Design review of the part built by this model. Coordinates are the model's own, in mm. A direction names the side the tool comes from. Coordinates: 2 decimals unless noted, no trailing zeros. Write each loop counter-clockwise with the first axis right and the second up, starting at its lowest first coordinate (ties: lowest second). Pieces come first, ordered by that corner, then holes.
Q1. For L1, parallel to Y at x = 37, z = 4.75; L2, parallel to Z at x = 2.5, y = 39; L3, parallel to X at y = 6.5, z = 3.25, list the stretches that pass through material, from the lowest coordinate up.
Q2. For faces 3 (the cylindrical face through (28, 9.1, 14)), 4 (the flat face through (36, 22, 13)), list the 3-axis set-ups (+Z, -Z, +X, -X, +Y, -Y) from which the entire face can be reached by the end or side of a thin tool; tool diameter is ignored.
Q3. The part is to be moulded in two halves that separate along Z. For faces 1 (the flat face through (21, 36, 2)), 2 (the flat face through (43, 22, 14)), say which applies: released by +Z, released by -Z, zero draft, split by the parting line, or undercut.
Q4. Take a section at C-C, the plane x = 37. Write out the cut boundary in (y, z).
Q5. For pin 1 Ø22.5 at (x, y) = (21.5, 21.5) entering from +Z, flat-tipped, find the tip position at first contact; note if it passes through.
Q6. Take a section at B-B, the plane x = 21.5. Write out the cut boundary in (y, z), plus the area to 3 significant figures.
Q7. Take a section at A-A, the plane z = 5.5. Write out the cut boundary in (x, y).
Solid Edge part; units mm, degrees
sketch "Sketch1" plane through (0, 0, 0) normal (0, 0, 1) x (1, 0, 0)
  line L0 (7, 0) -> (36, 0)
  arc A0 (36, 0) -> (43, 7) centre (36, 7) ccw
  line L1 (43, 7) -> (43, 36)
  arc A1 (43, 36) -> (36, 43) centre (36, 36) ccw
  line L2 (36, 43) -> (7, 43)
  arc A2 (7, 43) -> (0, 36) centre (7, 36) ccw
  line L3 (0, 36) -> (0, 7)
  arc A3 (7, 0) -> (0, 7) centre (7, 7) cw
  circle A4 centre (21.5, 21.5) radius 14
  circle A5 centre (6, 37) radius 1.7
  circle A6 centre (37, 37) radius 1.7
  circle A7 centre (6, 6) radius 1.7
  circle A8 centre (37, 6) radius 1.7
extrude "Protrusion1" add sketch "Sketch1" along normal blind 2
sketch "Sketch2" plane through (21.5, 21.5, 2) normal (0, 0, 1) x (1, 0, 0)
  circle A0 centre (-15.5, -15.5) radius 3.5
  circle A1 centre (-15.5, 15.5) radius 3.5
  circle A2 centre (15.5, 15.5) radius 3.5
  circle A3 centre (15.5, -15.5) radius 3.5
  circle A4 centre (-15.5, 15.5) radius 1.7
  circle A5 centre (15.5, 15.5) radius 1.7
  circle A6 centre (-15.5, -15.5) radius 1.7
  circle A7 centre (15.5, -15.5) radius 1.7
extrude "ExtrudedProtrusion_2" add sketch "Sketch2" along normal blind 11
mirror "Mirror1" about plane through (21.5, 21.5, 7.5) normal (0, 0, -1) of "Protrusion1"
Responses:
1. L1: y = 2.5 to 4.3, 7.7 to 9.5, 33.5 to 35.3, 38.7 to 40.5
1. L2: z = 0 to 2, 13 to 15
1. L3: x = 2.54 to 4.38, 7.62 to 9.46, 33.54 to 35.38, 38.62 to 40.46
2. face 3: +Z, -Z
2. face 4: none
3. face 1: undercut
3. face 2: zero draft
4. outline: (0.07, 0) - (4.3, 0) - (4.3, 15) - (0.07, 15) - (0.07, 13) - (2.5, 13) - (2.5, 2) - (0.07, 2) - close; (7.7, 0) - (35.3, 0) - (35.3, 15) - (7.7, 15) - close; (38.7, 0) - (42.93, 0) - (42.93, 2) - (40.5, 2) - (40.5, 13) - (42.93, 13) - (42.93, 15) - (38.7, 15) - close; hole (9.5, 2) - (33.5, 2) - (33.5, 13) - (9.5, 13) - close
5. pin 1: passes through
6. outline: (0, 0) - (7.5, 0) - (7.5, 2) - (0, 2) - close; (0, 13) - (7.5, 13) - (7.5, 15) - (0, 15) - close; (35.5, 0) - (43, 0) - (43, 2) - (35.5, 2) - close; (35.5, 13) - (43, 13) - (43, 15) - (35.5, 15) - close
6. area: 60.0 mm2
7. outline: circle Ø7 at (6, 6); circle Ø7 at (6, 37); circle Ø7 at (37, 6); circle Ø7 at (37, 37); hole circle Ø3.4 at (6, 6); hole circle Ø3.4 at (6, 37); hole circle Ø3.4 at (37, 6); hole circle Ø3.4 at (37, 37)
